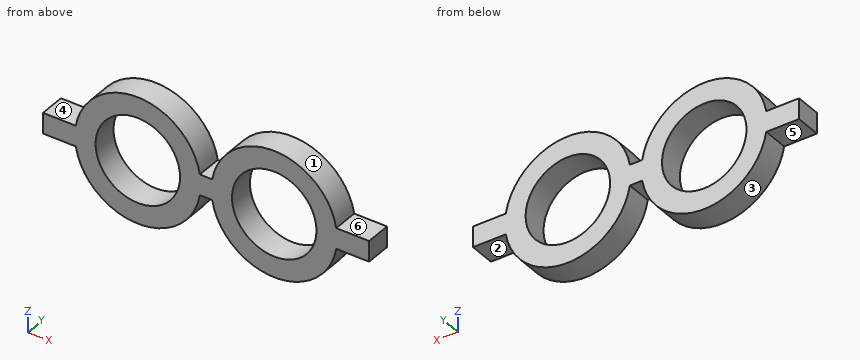
from build123d import *

# Parameters (mm, degrees)
F0_R     = 8.2
F1_DEPTH = 5


with BuildPart() as f1:
    # F0 (on Front) → F1 (new body)
    with BuildSketch(Plane.XZ):
        with BuildLine():
            Line((-18.4, -2), (-12.034949, -2))
            ThreePointArc((-12.034949, -2), (0, -12.2), (12.034949, -2))
            Line((12.034949, -2), (14.427051, -2))
            ThreePointArc((14.427051, -2), (26.462, -12.2), (38.496949, -2))
            Line((38.496949, -2), (44.862, -2))
            Line((44.862, -2), (44.862, 2))
            Line((44.862, 2), (38.496949, 2))
            ThreePointArc((38.496949, 2), (26.462, 12.2), (14.427051, 2))
            Line((14.427051, 2), (12.034949, 2))
            ThreePointArc((12.034949, 2), (0, 12.2), (-12.034949, 2))
            Line((-12.034949, 2), (-18.4, 2))
            Line((-18.4, 2), (-18.4, -2))
        make_face()
        Circle(F0_R, mode=Mode.SUBTRACT)
        with Locations((26.462, 0)):
            Circle(F0_R, mode=Mode.SUBTRACT)
    extrude(amount=F1_DEPTH)


solid = f1.part
Work out the finished part from the listing and answer in its coordinate system (mm). Face numbers are marked on the shaded views. A direction names the side the tool comes from. Give positions to 0.01 mm unless a question says otherwise; leave off trailing zeros. Write each loop counter-clockwise with the first axis right and the second up, starting at its lowest first coordinate (ties: lowest second). Pieces come first, ordered by that corner, then holes.
Q1. A tool of negligible diameter and unlimited length cuts with its end or side. For the marked faces 4, 5 and 6, from which of +Z, -Z, +X, -X, +Y, -Y can it reach the whole face along a straight path? Write none if from no direction.
Answer:
face 4: +Z, -X, +Y, -Y
face 5: -Z, -X, +Y, -Y
face 6: +Z, +X, +Y, -Y
Q2. Given pin 1 (2 mm diameter, centred on y = -1, z = 4.5, fed in from +X); pin 2 (1 mm diameter, centred on x = 28, y = -0.5, fed in from +Z); pin 3 (3 mm diameter, centred on x = 30, y = -2.5, fed in from +Z); pin 4 (8 mm diameter, centred on x = -1, z = -0.5, fed in from +Y), each flat-ended and moving along its own axis, determine where each tip first touches the part or whether it passes through.
Answer:
pin 1: stops at x = 38.15
pin 2: stops at z = 12.16
pin 3: stops at z = 12.03
pin 4: passes through
Q3. Straight lines are drawn through the part: L1, parallel to X at y = -1.1, z = 4.75; L2, parallel to X at y = -2.55, z = -1.25; L3, parallel to X at y = -2.85, z = -7.5. For each, find the intervals that lie inside material, in ascending order.
Answer:
L1: x = -11.24 to -6.68, 6.68 to 11.24, 15.22 to 19.78, 33.15 to 37.7
L2: x = -18.4 to -8.1, 8.1 to 18.36, 34.57 to 44.86
L3: x = -9.62 to -3.32, 3.32 to 9.62, 16.84 to 23.15, 29.78 to 36.08
Q4. The part is cut by section B-B on z = 0. Give the vertices of the cut face in (x, y), and give its area (3 significant figures).
Answer:
outline: (-18.4, -5) - (-8.2, -5) - (-8.2, 0) - (-18.4, 0) - close; (8.2, -5) - (18.26, -5) - (18.26, 0) - (8.2, 0) - close; (34.66, -5) - (44.86, -5) - (44.86, 0) - (34.66, 0) - close
area: 152 mm2
Q5. The part is cut by section A-A on y = -1.7. Give the vertices of the cut face in (x, z), and give its area (3 significant figures).
Answer:
outline: (-18.4, -2) - (-12.03, -2) arc R12.2 ccw to (12.03, -2) - (14.43, -2) arc R12.2 ccw to (38.5, -2) - (44.86, -2) - (44.86, 2) - (38.5, 2) arc R12.2 ccw to (14.43, 2) - (12.03, 2) arc R12.2 ccw to (-12.03, 2) - (-18.4, 2) - close; hole circle Ø16.4 at (0, 0); hole circle Ø16.4 at (26.46, 0)
area: 571 mm2
Q6. For a pull along X with two mould halves and no side action, classify the marked faces 1, 2 and 3 as released by +X, released by -X, zero draft, split by the parting line, or undercut.
Answer:
face 1: undercut
face 2: zero draft
face 3: undercut
Q7. The part is cut by section C-C on x = 0. Give the vertices of the cut face in (y, z).
Answer:
outline: (-5, -12.2) - (0, -12.2) - (0, -8.2) - (-5, -8.2) - close; (-5, 8.2) - (0, 8.2) - (0, 12.2) - (-5, 12.2) - close
Q8. The part is cut by section D-D on z = 9.25. Give the vertices of the cut face in (x, y).
Answer:
outline: (-7.95, -5) - (7.95, -5) - (7.95, 0) - (-7.95, 0) - close; (18.51, -5) - (34.42, -5) - (34.42, 0) - (18.51, 0) - close
